Part model, mm, in its own coordinate system. A direction names the side the tool comes from. Give positions to 0.01 mm unless a question says otherwise; leave off trailing zeros. Order: outer loops, then holes, each group sorted by start corner. A loop starts at its lowest first (then second) coordinate and runs counter-clockwise, first axis right, second up. Notation, with made-up numbers: M 8.25,66.25 L 54.25,66.25 A22 cw 54.25,100.25 Z; hole C -27.5,56.25 d5. An arc over 180 degrees is marked long. Answer as a JSON object with one key per item and string values.
from build123d import *

# Parameters (mm, degrees)
PLATE_DEPTH           = 3
SKETCH2_R             = 6
MOUNT_POSTS_DEPTH     = 22
SKETCH3_R             = 4.25
MOUNT_CBORE_DEPTH     = 19.5
F_8_CLEARANCE_HOLE1_D = 4.4958
FILLET1_R             = 1.5
SKETCH7_R             = 1.9
TERMINAL_STRIP_DEPTH  = 159.962259672
CHAMFER1_SIZE         = 3
CHAMFER2_SIZE         = 1
FILLET3_R             = 1.5
CORNERS_R             = 5


# Some blends are built 0.0001 mm under size
with BuildPart() as part:
    # Sketch1 → plate (new body)
    with BuildSketch(Plane(origin=(0, 0, 0), x_dir=(1, 0, 0), z_dir=(0, 1, 0))):
        Polygon((0, 0), (83, 0), (83, -12), (121, -12), (121, 88), (96, 88), (96, 98), (0, 98), align=None)
    extrude(amount=PLATE_DEPTH)

    # Sketch2 → mount posts (add)
    with BuildSketch(Plane(origin=(0, 3, 0), x_dir=(1, 0, 0), z_dir=(0, 1, 0))):
        with Locations(Location((75, 73.75, 0), (0, 0, 270))):
            Circle(SKETCH2_R)
        with Locations(Location((75, 12.25, 0), (0, 0, 270))):
            Circle(SKETCH2_R)
    extrude(amount=-MOUNT_POSTS_DEPTH)

    # Sketch3 → mount cbore (cut)
    with BuildSketch(Plane(origin=(0, 3, 0), x_dir=(1, 0, 0), z_dir=(0, 1, 0))):
        with Locations(Location((75, 73.75, 0), (0, 0, 270))):
            Circle(SKETCH3_R)
        with Locations(Location((75, 12.25, 0), (0, 0, 270))):
            Circle(SKETCH3_R)
    extrude(amount=-MOUNT_CBORE_DEPTH, mode=Mode.SUBTRACT)

    # #8 Clearance Hole1 (through all)
    with Locations(Plane(origin=(0, -16.5, 0), x_dir=(1, 0, 0), z_dir=(0, 1, 0))):
        with Locations((75, 73.75), (75, 12.25)):
            Hole(F_8_CLEARANCE_HOLE1_D / 2)

    # Sketch8 → foot (revolve)
    with BuildSketch(Plane(origin=(0, 0, -43), x_dir=(1, 0, 0), z_dir=(0, 0, -1)), mode=Mode.PRIVATE) as foot_sk:
        Polygon((45.25, 0), (46.85, 0), (45.1, 29), (43.5, 29), align=None)
    revolve(foot_sk.sketch.rotate(Axis((40, 0, -43), (0, -1, 0)), 90), axis=Axis((40, 0, -43), (0, -1, 0)))

    # Fillet1
    fillet1_edges = [part.edges().sort_by_distance(p)[0] for p in [
        (40, 0, -48.25),
        (40, 0, -49.85),
    ]]
    fillet(fillet1_edges, radius=FILLET1_R)

    # Sketch7 → terminal strip (cut, through all)
    with BuildSketch(Plane(origin=(0, 3, 0), x_dir=(1, 0, 0), z_dir=(0, 1, 0))):
        with Locations(Location((107.15, 37.9, 0), (0, 0, 270))):
            Circle(SKETCH7_R)
        with Locations(Location((107.15, -0.2, 0), (0, 0, 270))):
            Circle(SKETCH7_R)
        with BuildLine():
            Line((102.65, 9.325), (102.65, 28.375))
            ThreePointArc((102.65, 28.375), (107.15, 32.875), (111.65, 28.375))
            Line((111.65, 28.375), (111.65, 9.325))
            ThreePointArc((111.65, 9.325), (107.15, 4.825), (102.65, 9.325))
        make_face()
    extrude(amount=-TERMINAL_STRIP_DEPTH, mode=Mode.SUBTRACT)

    # Chamfer1
    # the kernel refuses this chamfer: 3 mm, written as the material it adds along each edge
    with BuildSketch(Plane(origin=(75, -16.5, -73.75), x_dir=(0, 0, 1), z_dir=(-1, 0, 0))) as chamfer1_piece_1_section:
        Polygon((4.25, CHAMFER1_SIZE), (4.25 - CHAMFER1_SIZE, 0), (4.25, 0), align=None)
    chamfer1_piece_1 = revolve(axis=Axis((75, -16.5, -73.75), (0, 1, 0)), mode=Mode.PRIVATE)
    chamfer1_piece_1 = chamfer1_piece_1 - Plane(origin=(75, -14.490807126, -73.75), x_dir=(-1, 0, 0), z_dir=(0, -1, 0)) * Cylinder(2.2479, 17, mode=Mode.PRIVATE)
    add(chamfer1_piece_1)
    with BuildSketch(Plane(origin=(75, -16.5, -12.25), x_dir=(0, 0, 1), z_dir=(-1, 0, 0))) as chamfer1_piece_2_section:
        Polygon((4.25, CHAMFER1_SIZE), (4.25 - CHAMFER1_SIZE, 0), (4.25, 0), align=None)
    chamfer1_piece_2 = revolve(axis=Axis((75, -16.5, -12.25), (0, 1, 0)), mode=Mode.PRIVATE)
    chamfer1_piece_2 = chamfer1_piece_2 - Plane(origin=(75, -14.490807126, -12.25), x_dir=(-1, 0, 0), z_dir=(0, -1, 0)) * Cylinder(2.2479, 18, mode=Mode.PRIVATE)
    add(chamfer1_piece_2)

    # Chamfer2
    chamfer2_edges = [part.edges().sort_by_distance(p)[0] for p in [
        (75, -19, -79.75),
        (75, -19, -18.25),
    ]]
    chamfer(chamfer2_edges, length=CHAMFER2_SIZE)

    # Fillet3
    fillet3_edges = [part.edges().sort_by_distance(p)[0] for p in [
        (75, 0, -79.75),
        (75, 0, -18.25),
    ]]
    fillet(fillet3_edges, radius=FILLET3_R)

    # corners
    corners_edges = [part.edges().sort_by_distance(p)[0] for p in [
        (0, 1.5, -98),
        (96, 1.5, -98),
        (96, 1.5, -88),
        (121, 1.5, -88),
        (121, 1.5, 12),
        (83, 1.5, 12),
        (83, 1.5, 0),
        (0, 1.5, 0),
    ]]
    fillet(corners_edges, radius=CORNERS_R - 0.0001)  # a hair under: the kernel refuses the full size


solid = part.part
1. Which spindle directions (+Z, -Z, +X, -X, +Y, -Y) get a long thin tool onto all of the face, cutting with end or side? Do faces 4 (the cylindrical face through (71.23, -5.13, -71.79)), 5 (the cylindrical face through (107.249, 1.521, -4.826)), 6 (the cylindrical face through (79.06, -9.63, -78.17)). Say none if no direction does.
Worked answers:
{"face 4": "+Y", "face 5": "+Y, -Y", "face 6": "-Y"}
2. Two-plate mould, pull along Z, no slides. Class faces 1 (the flat face through (41, 1, 0)), 2 (the cylindrical face through (77.246, -17.276, -12.349)), 3 (the cylindrical face through (1, 2, -96)): +Z half, -Z half, draft (parallel to the pull), parting line (faces both ways), or undercut.
Worked answers:
{"face 1": "+Z half", "face 2": "undercut", "face 3": "-Z half"}
3. Cut at D-D on z = -43. Give the cut face in (x, y).
Worked answers:
{"outline": "M 0,0 L 31.74,0 A1.5 cw 33.24,-1.41 L 34.9,-29 L 36.5,-29 L 34.85,-1.59 A1.5 cw 36.34,0 L 43.66,0 A1.5 cw 45.15,-1.59 L 43.5,-29 L 45.1,-29 L 46.76,-1.41 A1.5 cw 48.26,0 L 121,0 L 121,3 L 0,3 Z"}
4. Cut at A-A on z = -73.75. Give the cut face in (x, y).
Worked answers:
{"outline": "M 0,0 L 67.5,0 A1.5 cw 69,-1.5 L 69,-18 L 70,-19 L 72.75,-19 L 72.75,-15.5 L 70.75,-13.5 L 70.75,3 L 0,3 Z; M 77.25,-19 L 80,-19 L 81,-18 L 81,-1.5 A1.5 cw 82.5,0 L 121,0 L 121,3 L 79.25,3 L 79.25,-13.5 L 77.25,-15.5 Z"}
5. Cut at B-B on x = 107.15. Give the cut face in (y, z) (3 decimals).
Worked answers:
{"outline": "M 0,-88 L 3,-88 L 3,-39.8 L 0,-39.8 Z; M 0,-36 L 3,-36 L 3,-32.875 L 0,-32.875 Z; M 0,-4.825 L 3,-4.825 L 3,-1.7 L 0,-1.7 Z; M 0,2.1 L 3,2.1 L 3,12 L 0,12 Z"}
6. Probe line 1 along Z through (x, y) = (107, 1); line 2 along X through (y, z) = (-17.35, -73.75); line 3 along Y through (x, z) = (70, -19). List the from-to ranges inside material, lowest first.
Worked answers:
{"line 1": "z = -88 to -39.79, -36.01 to -32.87, -4.83 to -1.69, 2.09 to 12", "line 2": "x = 69 to 72.75, 77.25 to 81", "line 3": "y = 0 to 3"}
7. Cut at C-C on y = -11. Give the cut face in (x, z), plus the area to 3 significant figures.
Worked answers:
{"outline": "C 40,-43 d12.37; C 75,-73.75 d12; C 75,-12.25 d12; hole C 40,-43 d9.17; hole C 75,-73.75 d8.5; hole C 75,-12.25 d8.5", "area": "167 mm^2"}
8. Pin check, flat tips, straight feed: P1, Ø3.5, axis at x = 43.5, y = 2, coming from the +Z side; P2, Ø0.9, axis at x = 110.5, y = 1.5, coming from the -Z side; P3, Ø1, axis at y = -5, z = -74, coming from the -X side; P4, Ø6, axis at x = 39.5, z = -42, coming from the -Y side. Stop position of each tip, or through.
Worked answers:
{"P1": "stops at z = 0", "P2": "stops at z = -88", "P3": "stops at x = 69", "P4": "stops at y = -29"}
